CAD build for the part. Positions are in the model's coordinates, mm. A direction names the side the tool comes from. Give positions to 0.01 mm unless a question says otherwise; leave off trailing zeros. Write each loop counter-clockwise with the first axis right and the second up, starting at its lowest first coordinate (ties: lowest second). Pieces come first, ordered by that corner, then holes. Notation, with made-up numbers: (-11.5, 7.5) -> (5.5, 7.5) arc R19 cw to (5.5, 13.5) -> close; hole circle Ø9 at (-36, 46). An arc over 180 degrees is marked (long way). Answer in a Markdown table with one row per item. Add a question column.
```python
from build123d import *

# Parameters (mm, degrees)
EXTRUDE_1_DEPTH = 2.7


with BuildPart() as part:
    # 草图1 → 凸台-拉伸1 (new body)
    with BuildSketch(Plane(origin=(0, 0, 0), x_dir=(1, 0, 0), z_dir=(0, 1, 0))):
        with BuildLine():
            Line((-12.369316877, 7.141428429), (-16.887495374, 9.75))
            ThreePointArc((-16.887495374, 9.75), (-15.186446596, 12.232000645), (-13.123802868, 14.422752799))
            Line((-13.123802868, 14.422752799), (-10.768248507, 11.834053578))
            ThreePointArc((-10.768248507, 11.834053578), (14.922212592, 5.77300367), (0, -16))
            ThreePointArc((0, -16), (-0.5, -16.5), (0, -17))
            ThreePointArc((0, -17), (14.922212592, -38.77300367), (-10.768248507, -44.834053578))
            Line((-10.768248507, -44.834053578), (-13.123802868, -47.422752799))
            ThreePointArc((-13.123802868, -47.422752799), (-15.186446596, -45.232000645), (-16.887495374, -42.75))
            Line((-16.887495374, -42.75), (-12.369316877, -40.141428429))
            ThreePointArc((-12.369316877, -40.141428429), (-10.683653707, -39.844745078), (-9.202193277, -40.701924362))
            ThreePointArc((-9.202193277, -40.701924362), (10.872513333, -38.078233337), (0, -21))
            ThreePointArc((0, -21), (-4.5, -16.5), (0, -12))
            ThreePointArc((0, -12), (10.872513333, 5.078233337), (-9.202193277, 7.701924362))
            ThreePointArc((-9.202193277, 7.701924362), (-10.683653707, 6.844745078), (-12.369316877, 7.141428429))
        make_face()
    extrude(amount=EXTRUDE_1_DEPTH)


solid = part.part
```
Item 1: Slice it at D-D, the plane z = 15. List the corners of the cut face in (x, y), then the cut area to 3 significant figures.
Item 2: Slice it at B-B, the plane x = 5.5. List the corners of the cut face in (y, z).
Item 3: Slice it at A-A, the plane y = 0.65. List the corners of the cut face in (x, z), then the cut area to 3 significant figures.
Item 4: Mould opens along X. For faces 1 (the face through (-11.963, 1.331, -13.147)), 2 (the face through (-11.93, 1.33, 46.11)), 3 (the face through (-15.16, 1.331, 45.265)), 4 (the face through (2, 0, 19)) say: released by +X, released by -X, zero draft, split by the parting line, or undercut.
Item 5: Which spindle directions (+Z, -Z, +X, -X, +Y, -Y) get a long thin tool onto all of the face, cutting with end or side? Do faces 5 (the face through (-10.66, 1.33, -6.85)), 6 (the face through (-15.21, 1.33, -12.2)), 7 (the face through (-14.66, 1.331, 41.464)). Say none if no direction does.
Item 6: Slice it at C-C, the plane z = 33. List the corners of the cut face in (x, y).
Item 7: Drop flat-ended pins along their axis: pin 1 Ø1 at (x, y) = (-5, 2) entering from -Z; pin 2 Ø1.5 at (x, y) = (-12.5, 2) entering from -Z. Give the stop position or say it passes through.
Item 8: Probe L1, parallel to Z at x = 6.5, y = 2.65; L2, parallel to Z at x = -2.5, y = 2.35; L3, parallel to Z at x = 11, y = 2.15. List the from-to ranges inside material, lowest first. Write a range as from..to.
Answer key:
| question | item | result |
|---|---|---|
| 1 | outline | (-4.24, 0) -> (5.57, 0) -> (5.57, 2.7) -> (-4.24, 2.7) -> close |
| 1 | area | 26.5 mm² |
| 2 | outline | (0, -15.02) -> (2.7, -15.02) -> (2.7, -10.67) -> (0, -10.67) -> close; (0, 10.67) -> (2.7, 10.67) -> (2.7, 15.02) -> (0, 15.02) -> close; (0, 17.98) -> (2.7, 17.98) -> (2.7, 22.33) -> (0, 22.33) -> close; (0, 43.67) -> (2.7, 43.67) -> (2.7, 48.02) -> (0, 48.02) -> close |
| 3 | outline | (-16.89, -9.75) arc R19.5 ccw to (-13.12, -14.42) -> (-10.77, -11.83) arc R16 ccw (long way) to (0, 16) arc R0.5 cw to (0, 17) arc R16 ccw (long way) to (-10.77, 44.83) -> (-13.12, 47.42) arc R19.5 ccw to (-16.89, 42.75) -> (-12.37, 40.14) arc R2.5 ccw to (-9.2, 40.7) arc R12 cw (long way) to (0, 21) arc R4.5 ccw to (0, 12) arc R12 cw (long way) to (-9.2, -7.7) arc R2.5 ccw to (-12.37, -7.14) -> close |
| 3 | area | 537 mm² |
| 4 | face 1 | undercut |
| 4 | face 2 | undercut |
| 4 | face 3 | released by -X |
| 4 | face 4 | zero draft |
| 5 | face 5 | +Y, -Y |
| 5 | face 6 | -Z, -X, +Y, -Y |
| 5 | face 7 | -X, +Y, -Y |
| 6 | outline | (12, 0) -> (16, 0) -> (16, 2.7) -> (12, 2.7) -> close |
| 7 | pin 1 | stops at z = -15.35 |
| 7 | pin 2 | stops at z = -14.42 |
| 8 | L1 | z = -14.62..-10.09, 10.09..14.62, 18.38..22.91, 43.09..47.62 |
| 8 | L2 | z = -15.8..-11.74, 12.76..20.24, 44.74..48.8 |
| 8 | L3 | z = -11.62..-4.8, 4.8..11.62, 21.38..28.2, 37.8..44.62 |
